Input: part model. Units: mm. Frame: model coordinates. Face numbers are marked on the shaded views. A direction names the side the tool comes from. Round coordinates to 2 decimals unless told otherwise and drop trailing zeros. Loops run counter-clockwise (first coordinate to the right, second up) from the corner with the lowest first, then second, coordinate; pieces in that order, holes last. Notation, with made-up numbers: (42.5, -13) -> (51.5, -13) arc R33 cw to (51.5, 26) -> close; hole circle Ø7 at (28, -29.75). An arc over 180 degrees is marked (long way). Answer as a JSON object with one key per item and string values. Group by question number.
Item 1: Pin query (flat end, axial travel): pin 1 (5 mm diameter, centred on y = 13, z = 0, fed in from -X); pin 2 (6.5 mm diameter, centred on x = 45.2, z = 8.5, fed in from +Y); pin 3 (1.2 mm diameter, centred on x = -68, z = 9, fed in from +Y); pin 4 (20 mm diameter, centred on x = -18.75, y = 0, fed in from -Z). Return the tip coordinate at first contact, or that it passes through.
Item 2: Section query A-A on x = -18.75. Return loops of the section in (y, z).
Item 3: Section query B-B on z = -2.5. Return loops of the section in (x, y).
Item 4: Set-up query: the marked faces 4 and 5. Return all of +Z, -Z, +X, -X, +Y, -Y with unobstructed straight access to the full face (end or side cutting, diameter ignored); none if empty.
Item 5: Material intervals for line 1 (Z direction, x = 1, y = -28.5); line 2 (X direction, y = -5, z = -7.5); line 3 (X direction, y = -24, z = 6), sorted ascending. Write a range as [from, to].
Item 6: Section query D-D on z = 15. Return loops of the section in (x, y).
Item 7: Draft query along Y for the marked faces 1, 2 and 3. Return one class per face: released by +Y, released by -Y, zero draft, split by the parting line, or undercut.
Item 8: Section query C-C on y = 0. Return loops of the section in (x, z), and give its area (3 significant figures).
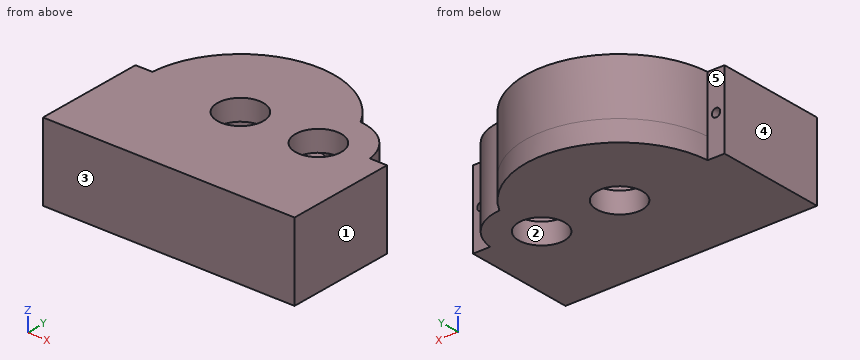
from build123d import *

# Parameters (mm, degrees)
BOSS_EXTRUDE2_DEPTH      = 27
SHELL5_DEPTH             = 17
BOSS_EXTRUDE3_START      = 10
BOSS_EXTRUDE3_DEPTH      = 10
SKETCH5_R                = 11
CUT_EXTRUDE2_DEPTH       = 87.360074687
BOSS_EXTRUDE4_DEPTH      = 37
BOSS_EXTRUDE5_DEPTH      = 3
BOSS_EXTRUDE5_DEPTH_BACK = 50
SKETCH10_R               = 2
CUT_EXTRUDE3_DEPTH       = 10


# Read off the part's stored shape, not the designer's step: Shell5
with BuildPart() as part:
    # Sketch1 → Boss-Extrude2 (new body)
    with BuildSketch(Plane.XY):
        with BuildLine():
            ThreePointArc((20.25, 22.449944321), (-63.75, 0), (20.25, -22.449944321))
            ThreePointArc((20.25, -22.449944321), (41.25, 0), (20.25, 22.449944321))
        make_face()
    extrude(amount=BOSS_EXTRUDE2_DEPTH)

    # Shell5 outline → Shell5 (cut)
    with BuildSketch(Plane.XY):
        with BuildLine():
            ThreePointArc((14.25, -11.66190379), (31.25, 0), (14.25, 11.66190379))
            ThreePointArc((14.25, 11.66190379), (-53.75, 0), (14.25, -11.66190379))
        make_face()
    extrude(amount=SHELL5_DEPTH, mode=Mode.SUBTRACT)

    # Sketch4 → Boss-Extrude3 (add)
    with BuildSketch(Plane(origin=(0, 0, 0), x_dir=(-1, 0, 0), z_dir=(0, 0, -1)).offset(BOSS_EXTRUDE3_START)):
        with BuildLine():
            ThreePointArc((-20.25, 22.449944321), (-41.25, 0), (-20.25, -22.449944321))
            ThreePointArc((-20.25, -22.449944321), (63.75, 0), (-20.25, 22.449944321))
        make_face()
    extrude(amount=-BOSS_EXTRUDE3_DEPTH)

    # Sketch5 → Cut-Extrude2 (cut, through all)
    with BuildSketch(Plane(origin=(0, 0, -10), x_dir=(-1, 0, 0), z_dir=(0, 0, -1))):
        with Locations((-18.75, 0)):
            Circle(SKETCH5_R)
        with Locations((18.75, 0)):
            Circle(SKETCH5_R)
    extrude(amount=-CUT_EXTRUDE2_DEPTH, mode=Mode.SUBTRACT)

    # Sketch8 → Boss-Extrude4 (add)
    with BuildSketch(Plane(origin=(0, 0, -10), x_dir=(-1, 0, 0), z_dir=(0, 0, -1))):
        with BuildLine():
            Line((-41.25, 0), (-41.25, -50))
            Line((-41.25, -50), (63.75, -50))
            Line((63.75, -50), (63.75, 0))
            ThreePointArc((63.75, 0), (30.368950039, -43.474130239), (-20.25, -22.449944321))
            ThreePointArc((-20.25, -22.449944321), (-35.181676725, -15.370426149), (-41.25, 0))
        make_face()
    extrude(amount=-BOSS_EXTRUDE4_DEPTH)

    # Sketch9 → Boss-Extrude5 (add, two sides: drawn at the far end of the back side and taken through both)
    with BuildSketch(Plane(origin=(0, 0, 0), x_dir=(1, 0, 0), z_dir=(0, 1, 0)).offset(-BOSS_EXTRUDE5_DEPTH_BACK)):
        Polygon((-71.75, -27), (-58.75, -27), (-58.75, -8.5), (-58.75, 10), (-71.75, 10), align=None)
        Polygon((36.25, -8.5), (36.25, 10), (49.25, 10), (49.25, -27), (36.25, -27), align=None)
    extrude(amount=BOSS_EXTRUDE5_DEPTH + BOSS_EXTRUDE5_DEPTH_BACK)

    # Sketch10 → Cut-Extrude3 (cut)
    with BuildSketch(Plane(origin=(0, 3, 0), x_dir=(1, 0, 0), z_dir=(0, 1, 0))):
        with Locations(Location((-67.699944321, -8.5, 0), (0, 0, 270))):
            Circle(SKETCH10_R)
        with Locations(Location((45.199944321, -8.5, 0), (0, 0, 90))):
            Circle(SKETCH10_R)
    extrude(amount=-CUT_EXTRUDE3_DEPTH, mode=Mode.SUBTRACT)


solid = part.part
Solved:
{
 "1": {"pin 1": "x = -62.51", "pin 2": "y = 3", "pin 3": "y = -7", "pin 4": "through"},
 "2": {"outline": "(-50, -10) -> (-11, -10) -> (-11, 0) -> (-35, 0) -> (-35, 17) -> (-11, 17) -> (-11, 27) -> (-50, 27) -> close; (11, -10) -> (45, -10) -> (45, 27) -> (11, 27) -> (11, 17) -> (35, 17) -> (35, 0) -> (11, 0) -> close"},
 "3": {"outline": "(-71.75, -50) -> (49.25, -50) -> (49.25, 3) -> (41.05, 3) arc R22.5 ccw to (20.25, 22.45) arc R45 ccw to (-63.65, 3) -> (-71.75, 3) -> close; hole circle Ø22 at (-18.75, 0); hole circle Ø22 at (18.75, 0)"},
 "4": {"face 4": "+Z, -Z, -X, +Y, -Y", "face 5": "+Z, -Z, -X, +Y"},
 "5": {"line 1": "[-10, 0], [17, 27]", "line 2": "[-71.75, -28.55], [-8.95, 8.95], [28.55, 49.25]", "line 3": "[-71.75, -44.23], [6.73, 49.25]"},
 "6": {"outline": "(-71.75, -50) -> (49.25, -50) -> (49.25, 3) -> (41.05, 3) arc R22.5 ccw to (20.25, 22.45) arc R45 ccw to (-63.65, 3) -> (-71.75, 3) -> close; hole (14.25, -11.66) arc R12.5 ccw (long way) to (14.25, 11.66) arc R35 ccw (long way) to start"},
 "7": {"face 1": "zero draft", "face 2": "undercut", "face 3": "released by -Y"},
 "8": {"outline": "(-71.75, -10) -> (-29.75, -10) -> (-29.75, 0) -> (-53.75, 0) -> (-53.75, 17) -> (-29.75, 17) -> (-29.75, 27) -> (-71.75, 27) -> close; (-7.75, -10) -> (7.75, -10) -> (7.75, 0) -> (-7.75, 0) -> close; (-7.75, 17) -> (7.75, 17) -> (7.75, 27) -> (-7.75, 27) -> close; (29.75, -10) -> (49.25, -10) -> (49.25, 27) -> (29.75, 27) -> (29.75, 17) -> (31.25, 17) -> (31.25, 0) -> (29.75, 0) -> close; hole circle Ø4 at (-67.7, 8.5); hole circle Ø4 at (45.2, 8.5)", "area": "2,130 mm²"}
}
